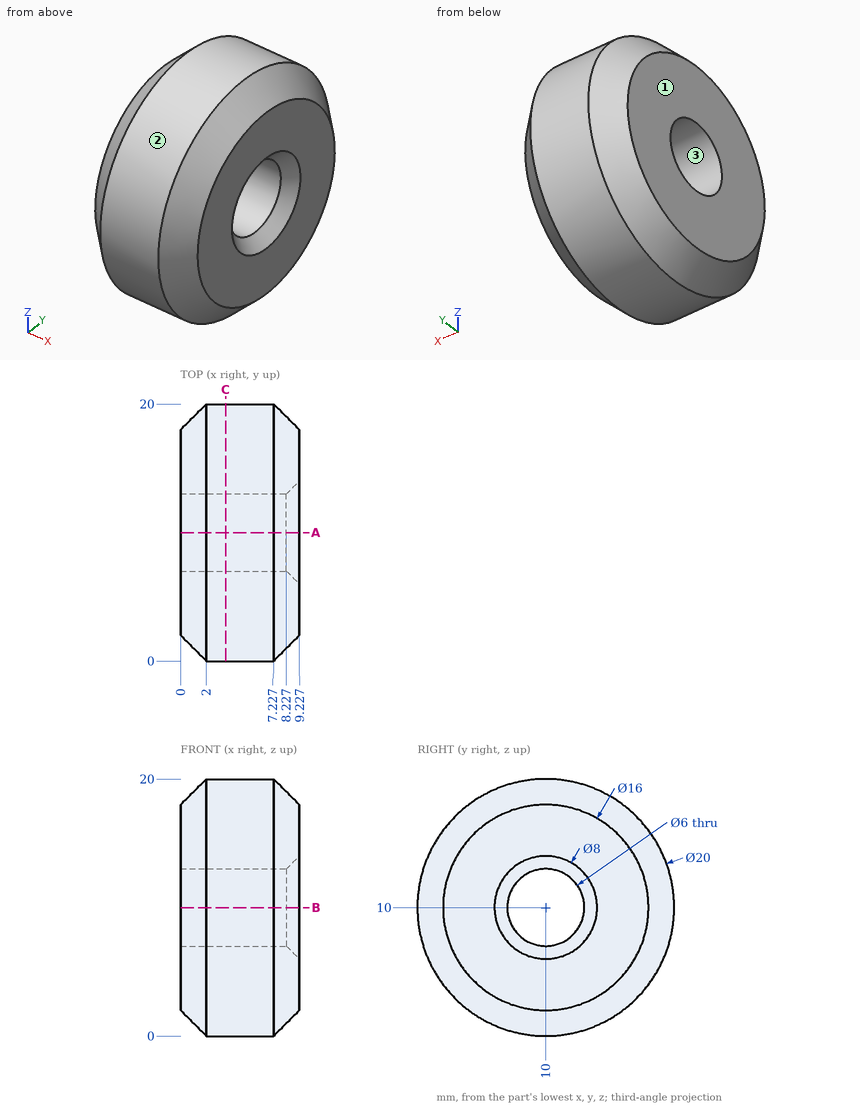
For this review, use the dimensioned drawing (mm, ordinates from the lowest corner) and the shaded views. Coordinates: 2 decimals unless noted, no trailing zeros. Write each loop counter-clockwise with the first axis right and the second up, starting at its lowest first coordinate (ties: lowest second). Pieces come first, ordered by that corner, then holes. Notation, with made-up numbers: (24.5, 88) - (67.5, 88) arc R18 cw to (67.5, 109) - close; hole circle Ø10 at (65, -7). An arc over 180 degrees is marked (long way). Answer in a Markdown table with one row per item. Add a question column.
Q1. Consider section C-C on x = 3.5. Give the boundary of the cut face in (y, z).
Q2. To check wall thickness, follow line 1 along Z through (x, y) = (5, 10); line 2 along Y through (x, z) = (7.75, 10.75) (1 decimal). State the ranges of each line that lie inside material, in increasing order. Write a range as from..to.
Q3. Draft analysis for pull direction Y (two halves, no side actions). For the marked faces 1, 2 and 3, state which applies: +Y half, -Y half, draft (parallel to the pull), parting line (faces both ways), or undercut.
Q4. Consider section A-A on y = 10. Give the boundary of the cut face in (x, z), then the cut area to 3 significant figures.
Q5. Clearance check with flat-ended pins moving along their axes: pin 1 (3 mm diameter, centred on x = 6, z = 7.5, fed in from +Y); pin 2 (1.5 mm diameter, centred on x = 7, y = 7, fed in from +Z); pin 3 (2 mm diameter, centred on x = 3.5, y = 3, fed in from -Z). State where each tip first meets the part, or that it passes through.
Answers below:
| question | item | result |
|---|---|---|
| 1 | outline | circle Ø20 at (10, 10); hole circle Ø6 at (10, 10) |
| 2 | line 1 | 0..7, 13..20 |
| 2 | line 2 | 0.6..7.1, 12.9..19.4 |
| 3 | face 1 | draft |
| 3 | face 2 | parting line |
| 3 | face 3 | undercut |
| 4 | outline | (0, 2) - (2, 0) - (7.23, 0) - (9.23, 2) - (9.23, 6) - (8.23, 7) - (0, 7) - close; (0, 13) - (8.23, 13) - (9.23, 14) - (9.23, 18) - (7.23, 20) - (2, 20) - (0, 18) - close |
| 4 | area | 120 mm² |
| 5 | pin 1 | y = 19.95 |
| 5 | pin 2 | z = 19.74 |
| 5 | pin 3 | z = 2 |
